Autodesk Inventor part; units mm, degrees
ref_plane "YZ Plane" through (0, 0, 0) normal (1, 0, 0) x (0, 1, 0)
ref_plane "XZ Plane" through (0, 0, 0) normal (0, 1, 0) x (-1, 0, 0)
ref_plane "XY Plane" through (0, 0, 0) normal (0, 0, 1) x (1, 0, 0)
sketch "Esboço1" plane through (0, 0, 0) normal (0, 0, 1) x (1, 0, 0)
  line L0 (-14.5, 7.5) -> (14.5, 7.5)
  line L1 (14.5, 7.5) -> (14.5, -7.5)
  line L2 (14.5, -7.5) -> (-14.5, -7.5)
  line L3 (-14.5, -7.5) -> (-14.5, 7.5)
  line L4 (-14.5, 7.5) -> (14.5, -7.5) construction
  line L5 (14.5, 7.5) -> (-14.5, -7.5) construction
  point P0 (0, 0)
  dimension "d0" = 29
  dimension "d1" = 15
extrude "Extrusão1" add sketch "Esboço1" along normal blind 25
sketch "Esboço2" plane through (-14.5, 7.5, 0) normal (0, 1, 0) x (1, 0, 0)
  line L0 (0, 0) -> (0, -25)
  line L1 (0, 0) -> (0, -9)
  line L2 (29, 0) -> (29, -25)
  line L3 (29, 0) -> (29, -9)
  line L4 (1.5, 0) -> (27.5, 0)
  line L5 (27.5, 0) -> (27.5, -9)
  line L6 (27.5, -9) -> (1.5, -9)
  line L7 (1.5, -9) -> (1.5, 0)
  line L8 (1.5, 0) -> (27.5, -9) construction
  line L9 (27.5, 0) -> (1.5, -9) construction
  line L10 (1.5, 0) -> (0, -9)
  line L11 (27.5, 0) -> (29, -9)
  line L12 (29, 0) -> (0, 0)
  line L13 (0, 0) -> (0, -25)
  line L14 (29, -25) -> (0, -25)
  line L15 (29, 0) -> (29, -25)
  point P0 (14.5, 0)
  point P1 (14.5, -4.5)
  dimension "d4" = 9
  dimension "d5" = 9
  dimension "d6" = 26
extrude "Extrusão2" cut sketch "Esboço2" against normal through all contours L12 L10 L0 | L12 L2 L11
sketch "Esboço3" plane through (0, 0, 25) normal (0, 0, 1) x (1, 0, 0)
  circle A0 centre (10, 0) radius 3
  circle A1 centre (-10, 0) radius 3
  line L0 (-13, -7.5) -> (-13, 7.5)
  line L1 (-7, 3) -> (-13, 3)
  line L2 (-13, 3) -> (-13, -3)
  line L3 (-13, -3) -> (-7, -3)
  line L4 (-7, -3) -> (-7, 3)
  line L5 (-7, 3) -> (-13, -3) construction
  line L6 (-13, 3) -> (-7, -3) construction
  line L7 (13, 3) -> (7, 3)
  line L8 (7, 3) -> (7, -3)
  line L9 (7, -3) -> (13, -3)
  line L10 (13, -3) -> (13, 3)
  line L11 (13, 3) -> (7, -3) construction
  line L12 (7, 3) -> (13, -3) construction
  line L13 (3, -1.5) -> (-3, -1.5)
  line L14 (-3, -1.5) -> (-3, -7.5)
  line L15 (-3, -7.5) -> (3, -7.5)
  line L16 (3, -7.5) -> (3, -1.5)
  line L17 (3, -1.5) -> (-3, -7.5) construction
  line L18 (-3, -1.5) -> (3, -7.5) construction
  line L19 (-14.5, -7.5) -> (14.5, -7.5)
  point P0 (0, 0)
  point P1 (0, -4.5)
  point P2 (-7, 0)
  point P3 (-13, 0)
  point P4 (7, 0)
  point P5 (13, 0)
  dimension "d9" = 6
  dimension "d10" = 6
  dimension "d11" = 10
  dimension "d12" = 10
  dimension "d13" = 6
  dimension "d14" = 6
  dimension "d15" = 0
extrude "Extrusão3" cut sketch "Esboço3" against normal blind 10 contours A0 | A0 L7 L10 | A0 L8 L7 | A1 | A1 L1 L4 | A1 L0 L1
sketch "Esboço4" plane through (-14.5, -7.5, 25) normal (-1, 0, 0) x (0, 0, 1)
  line L0 (-7, 12) -> (-10, 12)
  line L1 (-10, 12) -> (-10, 3)
  line L2 (-10, 3) -> (-7, 3)
  line L3 (-7, 3) -> (-7, 12)
  line L4 (-7, 12) -> (-10, 3) construction
  line L5 (-10, 12) -> (-7, 3) construction
  line L6 (-10, 7.5) -> (-10, 10.5)
  point P0 (-25, 7.5)
  point P1 (-8.5, 7.5)
  dimension "d18" = 3
  dimension "d19" = 9
  dimension "d20" = 0
extrude "Extrusão4" cut sketch "Esboço4" against normal blind 7.5
sketch "Esboço5" plane through (14.5, -7.5, 25) normal (1, 0, 0) x (0, 0, -1)
  line L0 (7, 3) -> (10, 3)
  line L1 (10, 3) -> (10, 12)
  line L2 (10, 12) -> (7, 12)
  line L3 (7, 12) -> (7, 3)
  line L4 (0, 7.5) -> (10, 7.5)
  line L5 (7, 3) -> (10, 12) construction
  line L6 (10, 3) -> (7, 12) construction
  line L7 (10, 4.5) -> (10, 7.5)
  point P0 (25, 7.5)
  point P1 (8.5, 7.5)
  dimension "d23" = 3
  dimension "d24" = 9
  dimension "d25" = 0
extrude "Extrusão5" cut sketch "Esboço5" against normal blind 7.5
sketch "Esboço6" plane through (0, 0, 25) normal (0, 0, 1) x (1, 0, 0)
  line L0 (-3, -7.5) -> (3, -7.5)
  line L1 (3, -7.5) -> (3, -1.5)
  line L2 (3, -1.5) -> (-3, -1.5)
  line L3 (-3, -1.5) -> (-3, -7.5)
  line L4 (-3, -7.5) -> (3, -1.5) construction
  line L5 (3, -7.5) -> (-3, -1.5) construction
  line L6 (-14.5, -7.5) -> (14.5, -7.5)
  line L7 (-3, -0.5) -> (3, -0.5)
  line L8 (3, -0.5) -> (3, 3.5)
  line L9 (3, 3.5) -> (-3, 3.5)
  line L10 (-3, 3.5) -> (-3, -0.5)
  line L11 (-3, -0.5) -> (3, 3.5) construction
  line L12 (3, -0.5) -> (-3, 3.5) construction
  point P0 (0, 0)
  point P1 (0, -4.5)
  point P2 (0, 1.5)
  dimension "d28" = 6
  dimension "d29" = 6
  dimension "d30" = 0
  dimension "d31" = 6
  dimension "d32" = 4
extrude "Extrusão6" cut sketch "Esboço6" against normal blind 5
sketch "Esboço8" plane through (0, 0, 20) normal (0, 0, 1) x (1, 0, 0)
  line L0 (3, -7.5) -> (-3, -7.5)
  point P0 (0, 0)
  point P1 (0, -5.5)
  point P2 (0, -7.5)
  dimension "d42" = 2
  dimension "d43" = 0
hole "Furo1" at (0, -5.5, 20) direction (0, 0, -1) diameter 3 end through all
sketch "Esboço9" plane through (0, 0, 0) normal (0, 0, -1) x (-1, 0, 0)
  circle A0 centre (0, -5.5) radius 1.5
  circle A1 centre (0, -5.5) radius 2.5
  line L0 (2.5, -5.5) -> (2.5, -7.5)
  line L1 (13, -7.5) -> (-13, -7.5)
  line L2 (-2.5, -5.5) -> (-2.5, -7.5)
  line L3 (2.5, -7.5) -> (-2.5, -7.5)
  point P0 (0, 0)
  point P1 (-1.5, -7.5)
  point P2 (1.5, -7.5)
  point P3 (-1.5, -7.5)
  dimension "d44" = 5
extrude "Extrusão7" cut sketch "Esboço9" against normal blind 1 contours A1 L1 | L0 L1 A1 | A1 L1 L2 picked at (0.0603, -7.3297)
sketch "Esboço10" plane through (0, 0, 0) normal (0, 0, -1) x (-1, 0, 0)
  line L0 (14.5, 1) -> (7.5, 1)
  line L1 (7.5, 1) -> (7.5, -5)
  line L2 (7.5, -5) -> (14.5, -5)
  line L3 (14.5, -5) -> (14.5, 1)
  line L4 (14.5, 1) -> (7.5, -5) construction
  line L5 (7.5, 1) -> (14.5, -5) construction
  line L6 (14.5, 7.5) -> (14.5, -7.5)
  line L7 (13, -7.5) -> (2.5, -7.5)
  line L8 (-7.5, 1) -> (-14.5, 1)
  line L9 (-14.5, 1) -> (-14.5, -5)
  line L10 (-14.5, -5) -> (-7.5, -5)
  line L11 (-7.5, -5) -> (-7.5, 1)
  line L12 (-7.5, 1) -> (-14.5, -5) construction
  line L13 (-14.5, 1) -> (-7.5, -5) construction
  line L14 (-14.5, -7.5) -> (-14.5, 7.5)
  line L15 (-2.5, -7.5) -> (-13, -7.5)
  point P0 (0, 0)
  point P1 (11, -2)
  point P2 (11, -5)
  point P3 (-11, -2)
  dimension "d47" = 7
  dimension "d48" = 6
  dimension "d49" = 0
  dimension "d50" = 2.5
  dimension "d51" = 7
  dimension "d52" = 6
  dimension "d53" = 0
  dimension "d54" = 2.5
extrude "Extrusão8" cut sketch "Esboço10" against normal blind 5
sketch "Esboço11" plane through (0, 0, 5) normal (0, 0, -1) x (-1, 0, 0)
  line L0 (15.3333, 1) -> (12.3333, 1)
  line L1 (12.3333, 1) -> (12.3333, -5)
  line L2 (12.3333, -5) -> (15.3333, -5)
  line L3 (15.3333, -5) -> (15.3333, 1)
  line L4 (13.8333, 1) -> (13.8333, -5)
  line L5 (15.3333, 1) -> (12.3333, -5) construction
  line L6 (12.3333, 1) -> (15.3333, -5) construction
  line L7 (-12.3333, 1) -> (-15.3333, 1)
  line L8 (-15.3333, 1) -> (-15.3333, -5)
  line L9 (-15.3333, -5) -> (-12.3333, -5)
  line L10 (-12.3333, -5) -> (-12.3333, 1)
  line L11 (-13.8333, -5) -> (-13.8333, 1)
  line L12 (-12.3333, 1) -> (-15.3333, -5) construction
  line L13 (-15.3333, 1) -> (-12.3333, -5) construction
  point P0 (0, 0)
  point P1 (13.8333, -2)
  point P2 (-13.8333, -2)
  dimension "d57" = 3
  dimension "d58" = 6
  dimension "d59" = 3
  dimension "d60" = 6
extrude "Extrusão9" cut sketch "Esboço11" against normal blind 7.5
sketch "Esboço12" plane through (0, 0, 15) normal (0, 0, 1) x (1, 0, 0)
  arc A0 (7, 0) -> (13, 0) centre (10, 0) ccw
  arc A1 (-13, 0) -> (-7, 0) centre (-10, 0) ccw
  point P0 (0, 0)
  dimension "d70" = 0
  dimension "d71" = 0
  dimension "d72" = 0
  dimension "d73" = 0
hole "Furo2" at (10, 0, 15) at (-10, 0, 15) direction (0, 0, -1) diameter 3 depth 0.998 tip angle 118
sketch "Esboço14" plane through (0, 0, 20) normal (0, 0, 1) x (1, 0, 0)
  line L0 (3, 3.5) -> (3, -0.5)
  line L1 (-3, 3.5) -> (3, 3.5)
  line L2 (-3, -0.5) -> (-3, 3.5)
  line L3 (3, -0.5) -> (-3, -0.5)
  point P0 (0, 0)
extrude "Extrusão11" cut sketch "Esboço14" against normal through all
properties part number "BLOCO DE CONTATO"
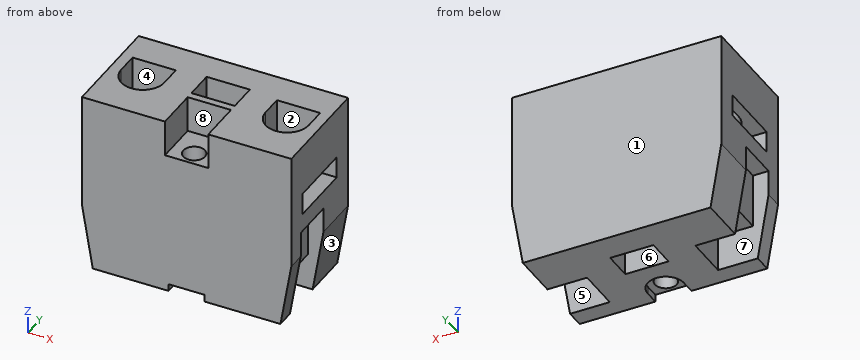
Source: CAD feature listing. Evaluate the final solid. Frame: model axes, mm. Face numbers are marked on the shaded views. A direction names the side the tool comes from. Give positions to 0.01 mm unless a question says otherwise; leave off trailing zeros. Write each loop counter-clockwise with the first axis right and the second up, starting at its lowest first coordinate (ties: lowest second). Pieces come first, ordered by that corner, then holes.
1. Material intervals for line 1 along X through (y, z) = (0, 14.2); line 2 along Y through (x, z) = (0, 14); line 3 along Y through (x, z) = (10, 14.25), sorted ascending.
2. First-contact query: pin 1 (2 mm diameter, centred on x = 0, y = -5.5, fed in from -Z); pin 2 (1.1 mm diameter, centred on x = -14, y = -2.5, fed in from -Z); pin 3 (8 mm diameter, centred on x = -6.5, y = 4.5, fed in from -Z); pin 4 (1.8 mm diameter, centred on y = -3.5, z = 8.5, fed in from -X). Flat tips, straight axial feed; report the tip coordinate or a pass-through.
3. Pull-direction query (Y, two-part tool) for the marked faces 1, 2 and 3; classes: +Y half, -Y half, draft (parallel to the pull), parting line (faces both ways), or undercut.
4. Access query for the marked faces 4, 5, 6, 7 and 8. Directions: +Z, -Z, +X, -X, +Y, -Y. A direction counts if a zero-diameter tool reaches every point of the face in a straight line with its end or side. Return the directions, or none.
5. Section query C-C (z = 18.75). Return the cut outline in (x, y), then the cut area to 3 significant figures.
6. Section query D-D (y = 6). Return the cut outline in (x, z), then the cut area to 4 significant figures.
7. Section query A-A (z = 23.25). Return the cut outline in (x, y), then the cut area to 3 significant figures.
8. Section query B-B (y = -2.5). Count the separate pieces of the cut face and the enclosed holes in it, then the cut area to 3 significant figures.
Output values:
1. line 1: x = -14.5 to -11.5, -8.5 to -3, 3 to 8.5, 11.5 to 14.5
1. line 2: y = -7.5 to -7, -4 to -0.5, 3.5 to 7.5
1. line 3: y = -7.5 to -1.5, 1.5 to 7.5
2. pin 1: passes through
2. pin 2: stops at z = 12.5
2. pin 3: stops at z = 0
2. pin 4: stops at x = -12.33
3. face 1: +Y half
3. face 2: undercut
3. face 3: draft
4. face 4: +Z
4. face 5: -Z, +X
4. face 6: +Z, -Z
4. face 7: -Z, -X
4. face 8: +Z, -Y
5. outline: (-14.5, -7.5) - (14.5, -7.5) - (14.5, 7.5) - (-14.5, 7.5) - close; hole (-13, 0) arc R3 ccw to (-7, 0) - (-7, 3) - (-13, 3) - close; hole (-3, -0.5) - (3, -0.5) - (3, 3.5) - (-3, 3.5) - close; hole circle Ø3 at (0, -5.5); hole (7, 0) arc R3 ccw to (13, 0) - (13, 3) - (7, 3) - close
5. area: 340 mm2
6. outline: (-14.5, 9) - (-13, 0) - (13, 0) - (14.5, 9) - (14.5, 25) - (-14.5, 25) - close
6. area: 711.5 mm2
7. outline: (-14.5, -7.5) - (-3, -7.5) - (-3, -1.5) - (3, -1.5) - (3, -7.5) - (14.5, -7.5) - (14.5, 7.5) - (-14.5, 7.5) - close; hole (-13, 0) arc R3 ccw to (-7, 0) - (-7, 3) - (-13, 3) - close; hole (-3, -0.5) - (3, -0.5) - (3, 3.5) - (-3, 3.5) - close; hole (7, 0) arc R3 ccw to (13, 0) - (13, 3) - (7, 3) - close
7. area: 311 mm2
8. separate pieces: 3
8. enclosed holes: 0
8. area: 501 mm2
